Autodesk Fusion 360 part; units mm, degrees
sketch "Sketch1" plane through (0, 0, 0) normal (0, 1, 0) x (1, 0, 0)
  line L0 (0, 0) -> (-33, 0)
  line L1 (0, 0) -> (33, 0)
  line L2 (-33, 0) -> (-38, 0)
  line L3 (33, 0) -> (38, 0)
  line L4 (-38, 0) -> (-38, -2.7218)
  line L5 (-36.2809, -6.4949) -> (-16.411, -23.773)
  line L6 (-13.1301, -25) -> (13.1301, -25)
  line L7 (38, 0) -> (38, -2.7218)
  line L8 (36.2809, -6.4949) -> (16.411, -23.773)
  arc A0 (-38, -2.7218) -> (-36.2809, -6.4949) centre (-33, -2.7218) ccw
  arc A1 (36.2809, -6.4949) -> (38, -2.7218) centre (33, -2.7218) ccw
  arc A2 (13.1301, -25) -> (16.411, -23.773) centre (13.1301, -20) ccw
  arc A3 (-16.411, -23.773) -> (-13.1301, -25) centre (-13.1301, -20) ccw
  line L9 (0, -4) -> (27.7062, -4)
  line L10 (33, -4) -> (33.0541, -4)
  line L11 (29.0185, -7.5092) -> (13.7863, -20.7546)
  arc A4 (13.1301, -21) -> (13.7863, -20.7546) centre (13.1301, -20) ccw
  line L12 (-13.1301, -21) -> (13.1301, -21)
  arc A5 (-13.7863, -20.7546) -> (-13.1301, -21) centre (-13.1301, -20) ccw
  line L13 (-29.0185, -7.5092) -> (-13.7863, -20.7546)
  line L14 (-33, -4) -> (-33.0541, -4)
  line L15 (0, -4) -> (-27.7062, -4)
  arc A6 (-27.7062, -4) -> (-29.0185, -7.5092) centre (-27.7062, -6) ccw
  arc A7 (29.0185, -7.5092) -> (27.7062, -4) centre (27.7062, -6) ccw
  dimension "d2" = 5
  dimension "d3" = 2
  dimension "d4" = 2
extrude "Extrude1" add sketch "Sketch1" along normal blind 9
sketch "Sketch2" plane through (0, 0, 0) normal (0, 0, -1) x (-1, 0, 0)
  line L0 (-38, 0) -> (38, 0)
  line L1 (38, 0) -> (38, 9)
  line L2 (38, 9) -> (-38, 9)
  line L3 (-38, 9) -> (-38, 0)
  line L4 (0, 0) -> (0, 9)
  line L5 (0, 4.5) -> (-33, 4.5)
  line L6 (0, 4.5) -> (33, 4.5)
  dimension "d7" = 33
  dimension "d8" = 33
hole "Hole1" at (33, 4.5, 0) at (-33, 4.5, 0) direction (0, 0, 1) diameter 3 depth 122 tip angle 180
sketch "Sketch3" plane through (0, 0, 25) normal (0, 0, 1) x (1, 0, 0)
  line L0 (-13.1301, 0) -> (13.1301, 0)
  line L1 (13.1301, 0) -> (13.1301, 9)
  line L2 (13.1301, 9) -> (-13.1301, 9)
  line L3 (-13.1301, 9) -> (-13.1301, 0)
  line L4 (0, 0) -> (0, 9)
  line L5 (0, 4.5) -> (-33, 4.5)
  line L6 (0, 4.5) -> (33, 4.5)
  dimension "d12" = 33
  dimension "d13" = 33
hole "Hole2" at (33, 4.5, 25) at (-33, 4.5, 25) direction (0, 0, -1) diameter 5 depth 20 tip angle 180
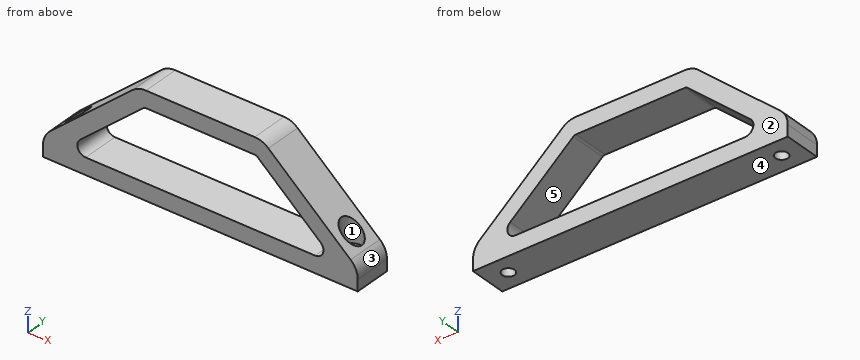
Could you check a few things on this model? Use its own coordinates, in mm. Face numbers are marked on the shaded views. A direction names the side the tool comes from. Round coordinates to 2 decimals unless told otherwise and drop trailing zeros. Order: outer loops, then holes, each group sorted by start corner. A loop starts at its lowest first (then second) coordinate and runs counter-clockwise, first axis right, second up.
(1) Imagine slicing it at D-D (y = 8). Write out the boundary of the cut face in (x, z), plus the area to 3 significant figures.
Response values:
outline: (-38, 0) - (38, 0) - (38, 2.72) arc R5 ccw to (36.28, 6.49) - (16.41, 23.77) arc R5 ccw to (13.13, 25) - (-13.13, 25) arc R5 ccw to (-16.41, 23.77) - (-36.28, 6.49) arc R5 ccw to (-38, 2.72) - close; hole (-29.02, 7.51) arc R2 ccw to (-27.71, 4) - (27.71, 4) arc R2 ccw to (29.02, 7.51) - (13.79, 20.75) arc R1 ccw to (13.13, 21) - (-13.13, 21) arc R1 ccw to (-13.79, 20.75) - close
area: 658 mm2
(2) Imagine slicing it at C-C (z = 10.75). Write out the boundary of the cut face in (x, y).
Response values:
outline: (-31.39, 0) - (-25.29, 0) - (-25.29, 9) - (-31.39, 9) - (-31.39, 6.41) arc R2.5 cw to (-31.39, 2.59) - close; (25.29, 0) - (31.39, 0) - (31.39, 2.59) arc R2.5 cw to (31.39, 6.41) - (31.39, 9) - (25.29, 9) - close
(3) If we mould it in two halves opening along X, with no side actions, what happens to the marked faces 1, 2 and 3? For each: released by +X, released by -X, zero draft, split by the parting line, or undercut.
Response values:
face 1: undercut
face 2: zero draft
face 3: released by +X
(4) Which directions (+Z, -Z, +X, -X, +Y, -Y) give clear straight access to the entire face, cutting with the end or side of a thin tool? Please do the marked faces 4 and 5.
Response values:
face 4: -Z, +X, -X, +Y, -Y
face 5: +Y, -Y
(5) I'm going to push flat-ended pins straight in: pin 1 (1 mm diameter, centred on y = 6, z = 5.5, fed in from +X); pin 2 (2.5 mm diameter, centred on x = 33, y = 4.5, fed in from +Z); pin 3 (2 mm diameter, centred on y = 4.5, z = 14, fed in from +X); pin 4 (2.5 mm diameter, centred on x = -32, y = 5.5, fed in from +Z). Where does each tip first touch, or does it pass through?
Response values:
pin 1: stops at x = 37.45
pin 2: passes through
pin 3: stops at x = 28.8
pin 4: stops at z = 11.3
(6) Imagine slicing it at B-B (x = 4). Write out the boundary of the cut face in (y, z), plus the area to 3 significant figures.
Response values:
outline: (0, 0) - (9, 0) - (9, 4) - (0, 4) - close; (0, 21) - (9, 21) - (9, 25) - (0, 25) - close
area: 72.0 mm2
(7) Imagine slicing it at A-A (y = 3.75). Count the separate pieces of the cut face and the enclosed holes in it, plus the area to 3 significant figures.
Response values:
separate pieces: 3
enclosed holes: 1
area: 591 mm2
(8) Please list where these lines run through material, in increasing order: line 1 along X through (y, z) = (4.5, 1.8); line 2 along Z through (x, y) = (1, 2); line 3 along Y through (x, z) = (-33, 7.5).
Response values:
line 1: x = -38 to -34.5, -31.5 to 31.5, 34.5 to 38
line 2: z = 0 to 4, 21 to 25
line 3: y = 0 to 2, 7 to 9
